Could you check a few things on this drawing? It's one solid part, dimensions in mm from its lowest x, y, z. A direction names the side the tool comes from. Give positions to 0.01 mm unless a question says otherwise; leave off trailing zeros. Write each loop counter-clockwise with the first axis right and the second up, starting at its lowest first coordinate (ties: lowest second). Pieces come first, ordered by that corner, then holes. Notation, with made-up numbers: (-5.75, -27) -> (16.25, -27) arc R18 ccw to (16.25, 7) -> close; hole circle Ø7 at (-16.5, 46.5). An arc over 180 degrees is marked (long way). Use CSV: the item, a comma, the result in double quotes. Start each with the question number.
(1) Suppose I cut it at A-A on y = 65. List the corners of the cut face in (x, z) for me, plus the area to 3 significant figures.
(2) Suppose I cut it at D-D on x = 2.5. List the corners of the cut face in (y, z) for me.
(3) Which directions (+Z, -Z, +X, -X, +Y, -Y) give clear straight access to the entire face, cutting with the end or side of a thin tool? Please do the marked faces 1 and 2.
(4) Suppose I cut it at B-B on x = 9. List the corners of the cut face in (y, z) for me, plus the area to 3 significant figures.
(5) Suppose I cut it at C-C on z = 3.5. List the corners of the cut face in (x, y) for me, plus the area to 3 significant figures.
(6) For pin 1 Ø1.5 at (y, z) = (46, 6) entering from -X; pin 2 Ø2 at (x, y) = (2.5, 30) entering from -Z, each with a flat end and sliding along its axis, tell me the tip position at first contact or that it passes through.
(7) I need wall thicknesses on L1, parallel to Y at x = 9, z = 7.4; L2, parallel to Y at x = 2.5, z = 5; L3, parallel to Z at x = 7.75, y = 15. Which ranges of each line are inside material? Lowest first, please. Write a range as [from, to].
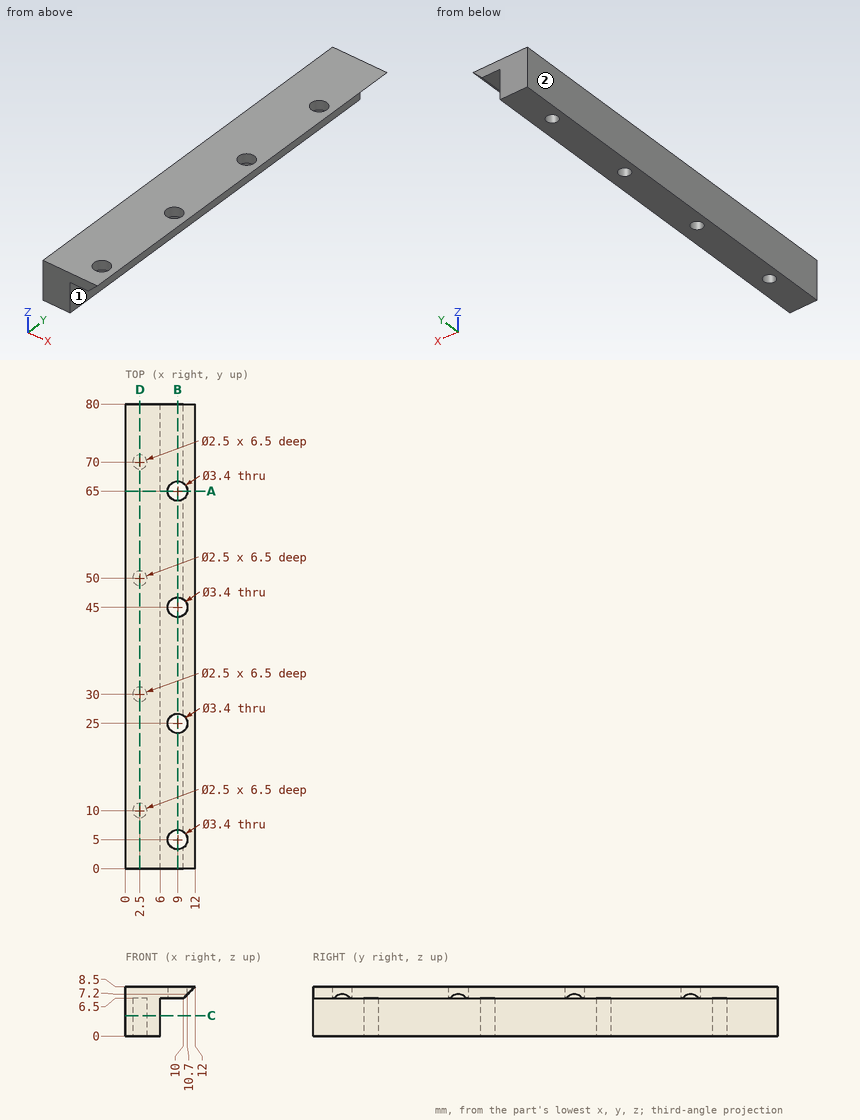
Geometry says:
1,outline,"(0, 0) -> (6, 0) -> (6, 6.5) -> (7.3, 6.5) -> (7.3, 8.5) -> (0, 8.5) -> close; (10.7, 7.2) -> (12, 8.5) -> (10.7, 8.5) -> close"
1,area,"54.4 mm²"
2,outline,"(0, 0) -> (8.75, 0) -> (8.75, 6.5) -> (11.25, 6.5) -> (11.25, 0) -> (28.75, 0) -> (28.75, 6.5) -> (31.25, 6.5) -> (31.25, 0) -> (48.75, 0) -> (48.75, 6.5) -> (51.25, 6.5) -> (51.25, 0) -> (68.75, 0) -> (68.75, 6.5) -> (71.25, 6.5) -> (71.25, 0) -> (80, 0) -> (80, 8.5) -> (0, 8.5) -> close"
3,face 1,"-Z, +X, +Y, -Y"
3,face 2,"+Z, -Z, -X, +Y, -Y"
4,outline,"(0, 6.5) -> (3.3, 6.5) -> (3.3, 8.5) -> (0, 8.5) -> close; (6.7, 6.5) -> (23.3, 6.5) -> (23.3, 8.5) -> (6.7, 8.5) -> close; (26.7, 6.5) -> (43.3, 6.5) -> (43.3, 8.5) -> (26.7, 8.5) -> close; (46.7, 6.5) -> (63.3, 6.5) -> (63.3, 8.5) -> (46.7, 8.5) -> close; (66.7, 6.5) -> (80, 6.5) -> (80, 8.5) -> (66.7, 8.5) -> close"
4,area,"133 mm²"
5,outline,"(0, 0) -> (6, 0) -> (6, 80) -> (0, 80) -> close; hole circle Ø2.5 at (2.5, 10); hole circle Ø2.5 at (2.5, 30); hole circle Ø2.5 at (2.5, 50); hole circle Ø2.5 at (2.5, 70)"
5,area,"460 mm²"
6,pin 1,"x = 0"
6,pin 2,"z = 6.5"
7,L1,"[0, 3.3], [6.7, 23.3], [26.7, 43.3], [46.7, 63.3], [66.7, 80]"
7,L2,"[0, 8.75], [11.25, 28.75], [31.25, 48.75], [51.25, 68.75], [71.25, 80]"
7,L3,"[6.5, 8.5]"
